CAD build for the part. Positions are in the model's coordinates, mm. Face numbers are marked on the shaded views. A direction names the side the tool comes from. Give positions to 0.01 mm unless a question says otherwise; leave off trailing zeros. Write each loop counter-clockwise with the first axis right and the second up, starting at its lowest first coordinate (ties: lowest second). Pieces come first, ordered by that corner, then holes. Notation, with made-up numbers: (8.5, 74.25) - (30.5, 74.25) arc R20 ccw to (30.5, 107.25) - close; hole circle Ø2 at (49, 29.25). An arc over 180 degrees is marked (long way). Answer as a JSON object with one key per item and string values.
from build123d import *

# Parameters (mm, degrees)
BOSS_EXTRUDE1_DEPTH = 7
FILLET1_R           = 2
SKETCH2_R           = 1.5
CUT_EXTRUDE1_DEPTH  = 7
SKETCH3_W           = 5
SKETCH3_H           = 7
BOSS_EXTRUDE2_DEPTH = 3
SKETCH4_R           = 1.5
CUT_EXTRUDE2_DEPTH  = 3
SKETCH5_R           = 1.5
CUT_EXTRUDE3_DEPTH  = 3


with BuildPart() as part:
    # Sketch1 → Boss-Extrude1 (new body)
    with BuildSketch(Plane(origin=(0, 0, 0), x_dir=(1, 0, 0), z_dir=(0, 1, 0))):
        Polygon((0, 0), (10, 0), (10, 3), (3, 3), (3, 36), (0, 36), align=None)
    extrude(amount=BOSS_EXTRUDE1_DEPTH)

    # Fillet1
    fillet1_edges = [part.edges().sort_by_distance(p)[0] for p in [
        (3, 3.5, -3),
    ]]
    fillet(fillet1_edges, radius=FILLET1_R)

    # Sketch2 → Cut-Extrude1 (cut)
    with BuildSketch(Plane(origin=(0, 0, -3), x_dir=(-1, 0, 0), z_dir=(0, 0, -1))):
        with Locations((-7.5, 3.5)):
            Circle(SKETCH2_R)
    extrude(amount=-CUT_EXTRUDE1_DEPTH, mode=Mode.SUBTRACT)

    # Sketch3 → Boss-Extrude2 (add)
    with BuildSketch(Plane.XY):
        with Locations((12.5, 3.5)):
            Rectangle(SKETCH3_W, SKETCH3_H)
    extrude(amount=-BOSS_EXTRUDE2_DEPTH)

    # Sketch4 → Cut-Extrude2 (cut)
    with BuildSketch(Plane(origin=(0, 0, -3), x_dir=(-1, 0, 0), z_dir=(0, 0, -1))):
        with Locations((-12.5, 3.5)):
            Circle(SKETCH4_R)
    extrude(amount=-CUT_EXTRUDE2_DEPTH, mode=Mode.SUBTRACT)

    # Sketch5 → Cut-Extrude3 (cut)
    with BuildSketch(Plane.ZY):
        with Locations((-32, 3.5)):
            Circle(SKETCH5_R)
    extrude(amount=-CUT_EXTRUDE3_DEPTH, mode=Mode.SUBTRACT)


solid = part.part
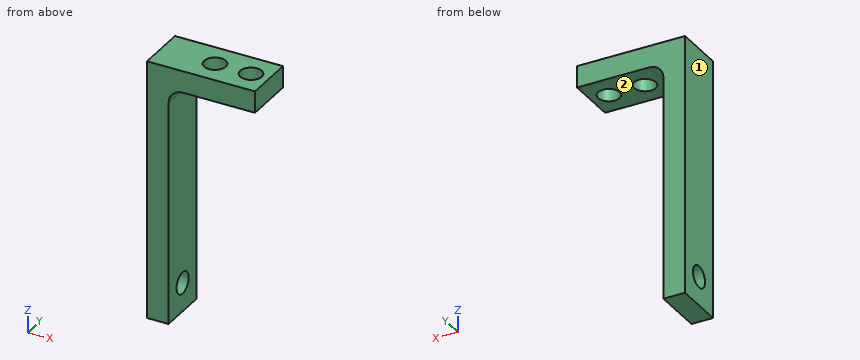
Item 1: Probe line 1 (X direction, y = 4.5, z = -1); line 2 (Y direction, x = 1.75, z = -32); line 3 (X direction, y = 1.75, z = -6.5). List the from-to ranges inside material, lowest first. Write a range as from..to.
Entries:
{"line 1": "0..6.38, 8.62..11.38, 13.62..15", "line 2": "0..2, 5..7", "line 3": "0..3"}
Item 2: Which spindle directions (+Z, -Z, +X, -X, +Y, -Y) get a long thin tool onto all of the face, cutting with end or side? Do the marked faces 1 and 2. Say none if no direction does.
Entries:
{"face 1": "+Z, -Z, -X, +Y, -Y", "face 2": "-Z, +X, +Y, -Y"}
Item 3: Cut at A-A (y = 3.5). Give the cut face in (x, z), and give its area (3 significant figures).
Entries:
{"outline": "(0, -36) - (3, -36) - (3, -33.5) - (0, -33.5) - close; (0, -30.5) - (3, -30.5) - (3, -5) arc R2 cw to (5, -3) - (6, -3) - (6, 0) - (0, 0) - close; (9, -3) - (11, -3) - (11, 0) - (9, 0) - close; (14, -3) - (15, -3) - (15, 0) - (14, 0) - close", "area": "118 mm2"}
Item 4: Cut at C-C (z = -31). Give the cut face in (x, y).
Entries:
{"outline": "(0, 0) - (3, 0) - (3, 2.38) - (0, 2.38) - close; (0, 4.62) - (3, 4.62) - (3, 7) - (0, 7) - close"}
Item 5: Cut at B-B (x = 1.75). Give the cut face in (y, z).
Entries:
{"outline": "(0, -36) - (7, -36) - (7, 0) - (0, 0) - close; hole circle Ø3 at (3.5, -32)"}
Item 6: Flat gauge pins, fed straight in: P1, Ø2, axis at x = 11, y = 2, coming from the -Z side; P2, Ø2, axis at y = 2, z = -24.5, coming from the +X side. Where does each tip first touch, or does it go through?
Entries:
{"P1": "z = -3", "P2": "x = 3"}
Item 7: Cut at D-D (x = 12.5). Give the cut face in (y, z).
Entries:
{"outline": "(0, -3) - (2, -3) - (2, 0) - (0, 0) - close; (5, -3) - (7, -3) - (7, 0) - (5, 0) - close"}
